For this review, use the dimensioned drawing (mm, ordinates from the lowest corner) and the shaded views. A direction names the side the tool comes from. Round coordinates to 2 decimals unless told otherwise and drop trailing zeros. Order: outer loops, then holes, each group sorted by start corner. A loop starts at its lowest first (then second) coordinate and runs counter-clockwise, first axis right, second up. Notation, with made-up numbers: M 85,3.5 L 136,3.5 A25 ccw 136,26.5 Z; hole C 70.5,9.5 d10. An arc over 180 degrees is marked long. One line per item, written item: value. Start each with the question number.
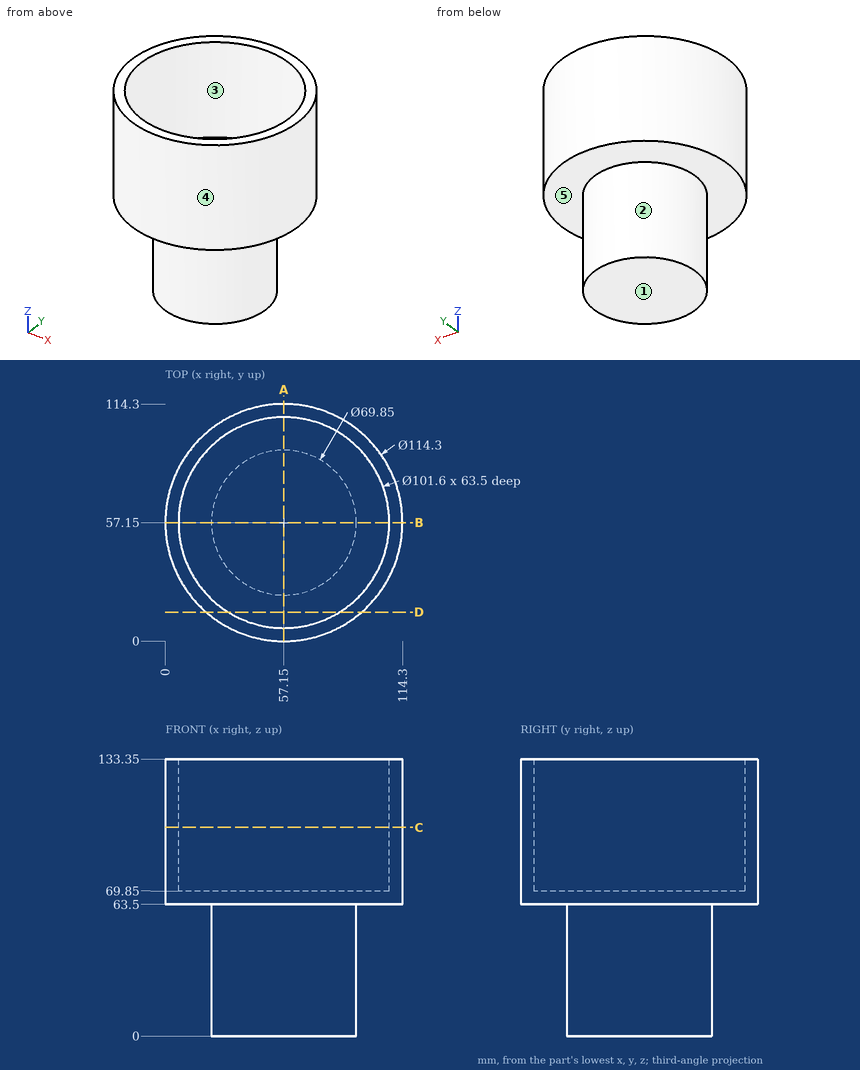
Item 1: The part is to be moulded in two halves that separate along X. For the marked faces 3, 4 and 5, say which applies: pulls with the +X half, pulls with the -X half, needs draft (parallel to the pull), parting line crosses it, or undercut.
Item 2: Consider section C-C, the plane z = 100.5. Give the boundary of the cut face in (x, y), then the cut area to 3 significant figures.
Item 3: Machinability: for the marked faces 1 and 2, which of the approach directions +Z, -Z, +X, -X, +Y, -Y give a long, thin tool a straight path to every point of the face, cutting with its end or side? Answer none if there is none.
Item 4: Consider section D-D, the plane y = 14. Give the boundary of the cut face in (x, z), then the cut area to 3 significant figures.
Item 5: Consider section A-A, the plane x = 57.15. Give the boundary of the cut face in (y, z) (3 decimals).
Item 6: Clearance check with flat-ended pins moving along their axes: P1, Ø1, axis at x = 69, z = 17.5, coming from the +Y side; P2, Ø12, axis at x = 71, z = 79.5, coming from the -Y side; P3, Ø2, axis at y = 52.5, z = 70, coming from the -X side. State where each tip first meets the part, or that it passes through.
Item 7: Wall thickness on L1, parallel to X at y = 57, z = 97; L2, parallel to Z at x = 16, y = 55: over which ranges is each line inside the solid? List them lowest first.
Computed:
1. face 3: undercut
1. face 4: parting line crosses it
1. face 5: needs draft
2. outline: C 57.15,57.15 d114.3; hole C 57.15,57.15 d101.6
2. area: 2,150 mm^2
3. face 1: -Z, +X, -X, +Y, -Y
3. face 2: -Z
4. outline: M 19.68,63.5 L 94.62,63.5 L 94.62,133.35 L 83.96,133.35 L 83.96,69.85 L 30.34,69.85 L 30.34,133.35 L 19.68,133.35 Z
4. area: 1,830 mm^2
5. outline: M 0,63.5 L 22.225,63.5 L 22.225,0 L 92.075,0 L 92.075,63.5 L 114.3,63.5 L 114.3,133.35 L 107.95,133.35 L 107.95,69.85 L 6.35,69.85 L 6.35,133.35 L 0,133.35 Z
6. P1: stops at y = 90.18
6. P2: stops at y = 0.54
6. P3: stops at x = 0.12
7. L1: x = 0 to 6.35, 107.95 to 114.3
7. L2: z = 63.5 to 69.85
